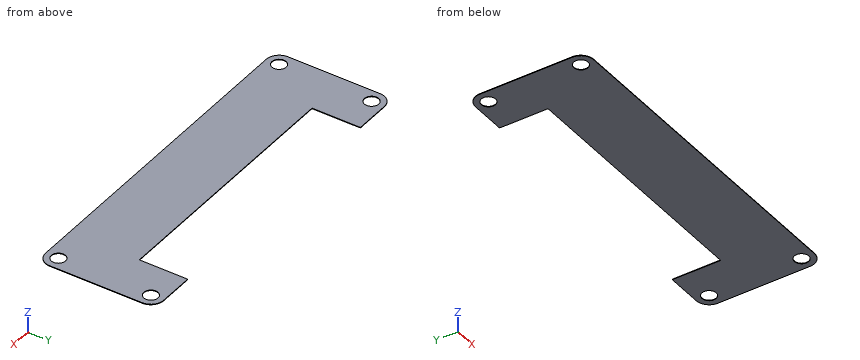
Autodesk Fusion 360 part; units mm, degrees
sketch "Sketch1" plane through (0, 0, 0) normal (0, 0, 1) x (1, 0, 0)
  line L0 (0, 0) -> (55, 0) construction
  line L1 (0, 0) -> (-55, 0) construction
  circle A0 centre (-57.5, 0) radius 2.5
  circle A1 centre (57.5, 0) radius 2.5
  line L2 (-57.5, -2.5) -> (-57.5, -30) construction
  line L3 (57.5, -2.5) -> (57.5, -30) construction
  circle A2 centre (57.5, -32.5) radius 2.5
  circle A3 centre (-57.5, -32.5) radius 2.5
  circle A4 centre (57.5, 0) radius 4.5
  circle A5 centre (57.5, -32.5) radius 4.5
  circle A6 centre (-57.5, -32.5) radius 4.5
  circle A7 centre (-57.5, 0) radius 4.5
  line L4 (-57.5, 4.5) -> (57.5, 4.5)
  line L5 (62, 0) -> (62, -32.5)
  line L6 (57.5, -37) -> (-57.5, -37)
  line L7 (-62, -32.5) -> (-62, 0)
  line L8 (45, -12.5) -> (-45, -12.5)
  line L9 (-45, -12.5) -> (-45, 12.5)
  line L10 (-45, 12.5) -> (45, 12.5)
  line L11 (45, 12.5) -> (45, -12.5)
  line L12 (45, -12.5) -> (-45, 12.5) construction
  line L13 (-45, -12.5) -> (45, 12.5) construction
  dimension "d1" = 55
  dimension "d2" = 55
  dimension "d4" = 27.5
  dimension "d5" = 27.5
  dimension "d6" = 5
  dimension "d7" = 5
  dimension "d8" = 9
  dimension "d9" = 9
  dimension "d10" = 9
  dimension "d11" = 9
  dimension "d12" = 90
  dimension "d13" = 25
extrude "Extrude1" add sketch "Sketch1" along normal blind 0.2 contours A4 | A4 A5 A6 A7 L4 L5 L6 L7 L8 L9 L11 | A5 | A6 | A7
equation "d1 = ( 110 / 2 ) * 1 mm"
equation "d2 = ( 110 / 2 ) * 1 mm"
Input: part model. Units: mm. Frame: model coordinates. Coordinates: 2 decimals unless noted, no trailing zeros. Order: outer loops, then holes, each group sorted by start corner. A loop starts at its lowest first (then second) coordinate and runs counter-clockwise, first axis right, second up. Notation, with made-up numbers: M 81.5,25.25 L 99.5,25.25 A21 ccw 99.5,49.25 Z; hole C 50.5,47.5 d10. An arc over 180 degrees is marked long. Answer in a Markdown table with one row per item.
(1) Section query B-B, the plane y = -11. Output: boundary loops of the cut face in (x, z), plus the area to 3 significant figures.
Numbers:
| item | result |
|---|---|
| outline | M -62,0 L -45,0 L -45,0.2 L -62,0.2 Z; M 45,0 L 62,0 L 62,0.2 L 45,0.2 Z |
| area | 6.80 mm^2 |
(2) Material intervals for line 1 (Y direction, x = -57.5, z = 0.1); line 2 (X direction, y = -10, z = 0.1); line 3 (Y direction, x = 11.5, z = 0.05), sorted ascending. Write a range as [from, to].
Numbers:
| item | result |
|---|---|
| line 1 | y = [-37, -35], [-30, -2.5], [2.5, 4.5] |
| line 2 | x = [-62, -45], [45, 62] |
| line 3 | y = [-37, -12.5] |
(3) Contact query for a flat-ended pin moving along its axis: pin 1 Ø3 at (x, y) = (-57.5, -32.5) entering from +Z. Output: stop coordinate, or through.
Numbers:
| item | result |
|---|---|
| pin 1 | passes through |
(4) Section query A-A, the plane z = 0.1. Output: boundary loops of the cut face in (x, y), plus the area to 3 significant figures.
Numbers:
| item | result |
|---|---|
| outline | M -62,-32.5 A4.5 ccw -57.5,-37 L 57.5,-37 A4.5 ccw 62,-32.5 L 62,0 A4.5 ccw 57.5,4.5 L 45,4.5 L 45,-12.5 L -45,-12.5 L -45,4.5 L -57.5,4.5 A4.5 ccw -62,0 Z; hole C -57.5,-32.5 d5; hole C -57.5,0 d5; hole C 57.5,-32.5 d5; hole C 57.5,0 d5 |
| area | 3,520 mm^2 |
(5) Section query C-C, the plane x = -9.5. Output: boundary loops of the cut face in (y, z), plus the area to 3 significant figures.
Numbers:
| item | result |
|---|---|
| outline | M -37,0 L -12.5,0 L -12.5,0.2 L -37,0.2 Z |
| area | 4.90 mm^2 |
